```python
from build123d import *

# Parameters (mm, degrees)
BOSS_EXTRUDE1_DEPTH      = 24
SKETCH2_R                = 2.75
CUT_EXTRUDE1_DEPTH       = 48
CUT_EXTRUDE2_DEPTH       = 21.5
CUT_EXTRUDE3_DEPTH       = 40.535585237
CHAMFER1_SIZE            = 2.3
CHAMFER1_OF_MIRROR1_SIZE = 2.3


with BuildPart() as part:
    # Sketch1 → Boss-Extrude1 (new, symmetric)
    with BuildSketch(Plane(origin=(0, 0, 0), x_dir=(0, 0, -1), z_dir=(1, 0, 0))):
        with BuildLine():
            Line((-17.25, 11.5), (-21.887338715, 7.895129733))
            ThreePointArc((-21.887338715, 7.895129733), (-25.75, 0), (-21.887338715, -7.895129733))
            Line((-21.887338715, -7.895129733), (-17.25, -11.5))
            Line((-17.25, -11.5), (17.25, -11.5))
            Line((17.25, -11.5), (17.25, 11.5))
            Line((17.25, 11.5), (-17.25, 11.5))
        make_face()
    extrude(amount=BOSS_EXTRUDE1_DEPTH, both=True)

    # Sketch2 → Cut-Extrude1 (cut)
    with BuildSketch(Plane(origin=(24, 0, 0), x_dir=(0, 0, -1), z_dir=(1, 0, 0))):
        with Locations((-15.75, 0)):
            Circle(SKETCH2_R)
        Polygon((17.25, 0), (-2.75, 11.5), (17.25, 11.5), align=None)
    extrude(amount=-CUT_EXTRUDE1_DEPTH, mode=Mode.SUBTRACT)

    # Sketch4 → Cut-Extrude2 (cut, symmetric)
    with BuildSketch(Plane(origin=(0, 0, 0), x_dir=(0, 0, -1), z_dir=(1, 0, 0))):
        with BuildLine():
            Line((17.25, -6.5), (17.25, 0))
            Line((17.25, 0), (-2.75, 11.5))
            Line((-2.75, 11.5), (-17.25, 11.5))
            Line((-17.25, 11.5), (-21.887338715, 7.895129733))
            ThreePointArc((-21.887338715, 7.895129733), (-25.75, 0), (-21.887338715, -7.895129733))
            Line((-21.887338715, -7.895129733), (-17.25, -11.5))
            Line((-17.25, -11.5), (-6.75, -11.5))
            Line((-6.75, -11.5), (-6.75, -9.5))
            Line((-6.75, -9.5), (-0.589824897, -9.5))
            Line((-0.589824897, -9.5), (3.25, -6.5))
            Line((3.25, -6.5), (17.25, -6.5))
        make_face()
    extrude(amount=CUT_EXTRUDE2_DEPTH, both=True, mode=Mode.SUBTRACT)

    # Sketch5 → Cut-Extrude3 (cut, through all)
    with BuildSketch(Plane(origin=(0, -6.5, 0), x_dir=(1, 0, 0), z_dir=(0, 1, 0))):
        with BuildLine():
            Line((6.5, 12.25), (12.5, 12.25))
            ThreePointArc((12.5, 12.25), (14.5, 10.25), (12.5, 8.25))
            Line((12.5, 8.25), (6.5, 8.25))
            ThreePointArc((6.5, 8.25), (4.5, 10.25), (6.5, 12.25))
        make_face()
    cut_extrude3 = extrude(amount=-CUT_EXTRUDE3_DEPTH, mode=Mode.SUBTRACT)

    # Chamfer1
    chamfer1_edges = [part.edges().sort_by_distance(p)[0] for p in [
        (4.5, -6.5, -10.25),
        (9.5, -6.5, -8.25),
        (14.5, -6.5, -10.25),
        (9.5, -6.5, -12.25),
    ]]
    chamfer(chamfer1_edges, length=CHAMFER1_SIZE)

    # Mirror1: Cut-Extrude3 across plane
    add(cut_extrude3.mirror(Plane(origin=(0, 0, 0), x_dir=(0, 0, 1), z_dir=(1, 0, 0))), mode=Mode.SUBTRACT)

    # Chamfer1 of Mirror1
    chamfer1_of_mirror1_edges = [part.edges().sort_by_distance(p)[0] for p in [
        (-4.5, -6.5, -10.25),
        (-9.5, -6.5, -8.25),
        (-14.5, -6.5, -10.25),
        (-9.5, -6.5, -12.25),
    ]]
    chamfer(chamfer1_of_mirror1_edges, length=CHAMFER1_OF_MIRROR1_SIZE)


solid = part.part
```
Work out the finished part from the listing and answer in its coordinate system (mm). A direction names the side the tool comes from. Round coordinates to 2 decimals unless told otherwise and drop trailing zeros. Write each loop counter-clockwise with the first axis right and the second up, starting at its lowest first coordinate (ties: lowest second). Pieces come first, ordered by that corner, then holes.
1) A cutting plane is placed at B-B on x = 7.5. Determine the outline of the cut face in (y, z), and give its area (3 significant figures).
2) A cutting plane is placed at D-D on z = 4. Determine the outline of the cut face in (x, y).
3) Consider probe 1 along X at (y, z) = (-7.25, 12.5); probe 2 along Y at (x, z) = (-23.05, 15.75); probe 3 along Y at (x, z) = (22, 15). Determine where each line is inside the solid, lowest interval first.
4) A cutting plane is placed at A-A on z = 11.5. Determine the outline of the cut face in (x, y).
5) A cutting plane is placed at C-C on y = 4. Determine the outline of the cut face in (x, z), and give its area (3 significant figures).
6) Determine the mould class of faces 1 (the face through (-22.73, 9.72, 19.54)), 2 (the face through (24, -2, 5)), 3 (the face through (15.1, -8.2, -10.3)), 4 (the face through (0.301, -8.021, -1.303)) for opening direction X: pulls with the +X half, pulls with the -X half, needs draft (parallel to the pull), parting line crosses it, or undercut.
7) Which of the six approach directions +Z, -Z, +X, -X, +Y, -Y give full straight-line access (tool end or side, diameter ignored) to faces 5 (the face through (0, -9.5, 4)), 6 (the face through (22.77, 9.72, 19.54)), 7 (the face through (-15.1, -8.2, -10.3)), 8 (the face through (0, -11.5, -4)), 9 (the face through (-9, -10, -12.25))?
8) Flat-ended cylindrical pins translate along their axes: P1, Ø0.8, axis at x = -8, y = -10, coming from the +Z side; P2, Ø5, axis at x = 1.5, z = 4.5, coming from the +Y side; P3, Ø7, axis at x = 1.5, z = -13, coming from the +Y side. Find the tip coordinate at first contact, or state that the pin passes through.
Entries:
1. outline: (-11.5, -17.25) - (-6.5, -17.25) - (-6.5, -14.55) - (-8.8, -12.25) - (-11.5, -12.25) - close; (-11.5, -8.25) - (-8.8, -8.25) - (-6.5, -5.95) - (-6.5, -3.25) - (-9.5, 0.59) - (-9.5, 6.75) - (-11.5, 6.75) - close
1. area: 70.5 mm2
2. outline: (-24, -11.5) - (24, -11.5) - (24, 11.5) - (21.5, 11.5) - (21.5, -9.5) - (-21.5, -9.5) - (-21.5, 11.5) - (-24, 11.5) - close
3. probe 1: x = -24 to -21.5, 21.5 to 24
3. probe 2: y = -11.5 to -2.75, 2.75 to 11.5
3. probe 3: y = -11.5 to -2.65, 2.65 to 11.5
4. outline: (-24, -11.5) - (-21.5, -11.5) - (-21.5, 11.5) - (-24, 11.5) - close; (21.5, -11.5) - (24, -11.5) - (24, 11.5) - (21.5, 11.5) - close
5. outline: (-24, -10.29) - (-21.5, -10.29) - (-21.5, 24.92) - (-24, 24.92) - close; (21.5, -10.29) - (24, -10.29) - (24, 24.92) - (21.5, 24.92) - close
5. area: 176 mm2
6. face 1: needs draft
6. face 2: pulls with the +X half
6. face 3: undercut
6. face 4: undercut
7. face 5: +Z, +Y
7. face 6: +Z, +X, -X, +Y
7. face 7: +Y
7. face 8: +Z, -Z, +X, -X, -Y
7. face 9: +Y, -Y
8. P1: stops at z = 6.75
8. P2: stops at y = -9.5
8. P3: stops at y = -6.5
